from build123d import *

# Parameters (mm, degrees)
BLANKSKE_W        = 21.75
BLANKSKE_H        = 2.55
BLANK_DEPTH       = 2.8
TOOTHCUTSIM_DEPTH = 23.077250735
TEETHCUTS_COUNT   = 18
TEETHCUTS_PITCH   = 1.25663706


with BuildPart() as part:
    # BlankSke → Blank (new body)
    with BuildSketch(Plane.XY):
        with Locations((10.875, 1.275)):
            Rectangle(BLANKSKE_W, BLANKSKE_H)
    extrude(amount=-BLANK_DEPTH)

    # TooCutSkeSim → ToothCutSim (cut, through all)
    with BuildSketch(Plane.XY):
        Polygon((0.177174148, 1.65), (-0.177174148, 1.65), (-0.513992203, 2.5754), (0.513992203, 2.5754), align=None)
    toothcutsim = extrude(amount=-TOOTHCUTSIM_DEPTH, mode=Mode.SUBTRACT)

    # TeethCuts: ToothCutSim ×18
    with Locations(*[(i * TEETHCUTS_PITCH, 0, 0) for i in range(1, TEETHCUTS_COUNT)]):
        add(toothcutsim, mode=Mode.SUBTRACT)


solid = part.part
Part model, mm, in its own coordinate system. A direction names the side the tool comes from. Give positions to 0.01 mm unless a question says otherwise; leave off trailing zeros. One line per question, with ' | ' between items.
1. Drill centre line: probe 1 along Y at (x, z) = (12.5, -1.6). Where is it in solid material? Low to high.
Filled in:
probe 1: 0 to 1.65
2. Which spindle directions (+Z, -Z, +X, -X, +Y, -Y) get a long thin tool onto all of the face, cutting with end or side? Do faces 1 (the face through (11, 1, 0)), 2 (the face through (17.936, 2.106, -1.38)). Say none if no direction does.
Filled in:
face 1: +Z, +X, -X, +Y, -Y | face 2: +Z, -Z, +Y
3. Pull direction X, two halves, no side cores. Call faces 3 (the face through (11, 0, -1)), 4 (the face through (10.971, 2.094, -1.38)), 5 (the face through (0, 1, -1)), 6 (the face through (18.511, 2.094, -1.38)): +X half, -X half, draft (parallel to the pull), parting line (faces both ways), or undercut.
Filled in:
face 3: draft | face 4: undercut | face 5: -X half | face 6: undercut
4. Band-saw the part on A-A on y = 1.85. Give the number of separate pieces and of enclosed holes in the cut face, then the cut area to 3 significant figures.
Filled in:
separate pieces: 18 | enclosed holes: 0 | area: 36.4 mm²
